from build123d import *

# Parameters (mm, degrees)
SKETCH1_W           = 70
SKETCH1_H           = 85
BOSS_EXTRUDE1_DEPTH = 70
SKETCH2_R           = 5
CUT_EXTRUDE1_DEPTH  = 20
SKETCH3_W           = 24.749109438
SKETCH3_H           = 45.30683744
CUT_EXTRUDE2_DEPTH  = 116.542200083
SKETCH4_R           = 3
CUT_EXTRUDE3_DEPTH  = 101.350635275
SKETCH6_W           = 18
SKETCH6_H           = 62.779044911
CUT_EXTRUDE4_DEPTH  = 116.542200083


with BuildPart() as part:
    # Sketch1 → Boss-Extrude1 (new body)
    with BuildSketch(Plane(origin=(0, 0, 0), x_dir=(1, 0, 0), z_dir=(0, 1, 0))):
        Rectangle(SKETCH1_W, SKETCH1_H)
    extrude(amount=BOSS_EXTRUDE1_DEPTH)

    # Sketch2 → Cut-Extrude1 (cut)
    with BuildSketch(Plane.XZ):
        with Locations(Location((0, 0, 0), (0, 0, 270))):
            Circle(SKETCH2_R)
    extrude(amount=-CUT_EXTRUDE1_DEPTH, mode=Mode.SUBTRACT)

    # Sketch3 → Cut-Extrude2 (cut, through all)
    with BuildSketch(Plane(origin=(0, 0, -42.5), x_dir=(-1, 0, 0), z_dir=(0, 0, -1))):
        with Locations((-35.374554719, 50.717680389)):
            Rectangle(SKETCH3_W, SKETCH3_H)
        with Locations((35.374554719, 50.717680389)):
            Rectangle(SKETCH3_W, SKETCH3_H)
    extrude(amount=-CUT_EXTRUDE2_DEPTH, mode=Mode.SUBTRACT)

    # Sketch4 → Cut-Extrude3 (cut, through all)
    with BuildSketch(Plane.ZY.offset(23)):
        with Locations(Location((-8.5, 50, 0), (0, 0, 270))):
            Circle(SKETCH4_R)
    extrude(amount=-CUT_EXTRUDE3_DEPTH, mode=Mode.SUBTRACT)

    # Sketch6 → Cut-Extrude4 (cut, through all)
    with BuildSketch(Plane(origin=(0, 0, -42.5), x_dir=(-1, 0, 0), z_dir=(0, 0, -1))):
        with Locations((0, 59.453784125)):
            Rectangle(SKETCH6_W, SKETCH6_H)
    extrude(amount=-CUT_EXTRUDE4_DEPTH, mode=Mode.SUBTRACT)


solid = part.part
The model under review builds one solid part; all positions refer to its coordinate system, in mm. A direction names the side the tool comes from. Coordinates: 2 decimals unless noted, no trailing zeros. Write each loop counter-clockwise with the first axis right and the second up, starting at its lowest first coordinate (ties: lowest second). Pieces come first, ordered by that corner, then holes. Notation, with made-up numbers: M 51.5,2.25 L 81.5,2.25 A21 ccw 81.5,6.25 Z; hole C 64.25,11.25 d10. An arc over 180 degrees is marked long. Put each result on its own line as item: value.
1) Clearance check with flat-ended pins moving along their axes: pin 1 Ø9.5 at (y, z) = (50, -8.5) entering from -X; pin 2 Ø16 at (x, z) = (0, 0) entering from -Y; pin 3 Ø9.5 at (x, z) = (-28, 11.5) entering from +Y; pin 4 Ø12.5 at (y, z) = (44, 20) entering from +X. State where each tip first meets the part, or that it passes through.
Computed:
pin 1: stops at x = -23
pin 2: stops at y = 0
pin 3: stops at y = 28.06
pin 4: stops at x = 23
2) Add section A-A on z = -8.5. Give the boundary of the cut face in (x, y), then the cut area to 3 significant figures.
Computed:
outline: M -35,0 L 35,0 L 35,28.06 L 23,28.06 L 23,47 L 9,47 L 9,28.06 L -9,28.06 L -9,47 L -23,47 L -23,28.06 L -35,28.06 Z; M -23,53 L -9,53 L -9,70 L -23,70 Z; M 9,53 L 23,53 L 23,70 L 9,70 Z
area: 2,970 mm2
3) Draft analysis for pull direction X (two halves, no side actions). For faces 1 (the flat face through (9, 49, -1)), 2 (the flat face through (35, 14, 1)), 3 (the flat face through (0, 27, -42.5)), state which applies: released by +X, released by -X, zero draft, split by the parting line, or undercut.
Computed:
face 1: undercut
face 2: released by +X
face 3: zero draft
4) For faces 4 (the flat face through (0, 20, 0)), 5 (the flat face through (-23, 49, -1)), 6 (the flat face through (29, 28.064, -1)), 7 (the flat face through (0, 28.064, -1)), list the 3-axis set-ups (+Z, -Z, +X, -X, +Y, -Y) from which the entire face can be reached by the end or side of a thin tool; tool diameter is ignored.
Computed:
face 4: -Y
face 5: +Z, -Z, -X, +Y
face 6: +Z, -Z, +X, +Y
face 7: +Z, -Z, +Y
5) Add section C-C on y = 37. Give the boundary of the cut face in (x, z), then the cut area to 3 significant figures.
Computed:
outline: M -23,-42.5 L -9,-42.5 L -9,42.5 L -23,42.5 Z; M 9,-42.5 L 23,-42.5 L 23,42.5 L 9,42.5 Z
area: 2,380 mm2
6) Wall thickness on probe 1 along Z at (x, y) = (15, 50); probe 2 along X at (y, z) = (41, 35); probe 3 along X at (y, z) = (7.5, 0): over which ranges is each line inside the solid? List them lowest first. Write a range as [from, to].
Computed:
probe 1: z = [-42.5, -11.5], [-5.5, 42.5]
probe 2: x = [-23, -9], [9, 23]
probe 3: x = [-35, -5], [5, 35]
7) Add section D-D on z = 10.5. Give the boundary of the cut face in (x, y), then the cut area to 3 significant figures.
Computed:
outline: M -35,0 L 35,0 L 35,28.06 L 23,28.06 L 23,70 L 9,70 L 9,28.06 L -9,28.06 L -9,70 L -23,70 L -23,28.06 L -35,28.06 Z
area: 3,140 mm2
8) Add section B-B on y = 50. Give the boundary of the cut face in (x, z), then the cut area to 3 significant figures.
Computed:
outline: M -23,-42.5 L -9,-42.5 L -9,-11.5 L -23,-11.5 Z; M -23,-5.5 L -9,-5.5 L -9,42.5 L -23,42.5 Z; M 9,-42.5 L 23,-42.5 L 23,-11.5 L 9,-11.5 Z; M 9,-5.5 L 23,-5.5 L 23,42.5 L 9,42.5 Z
area: 2,210 mm2
